Can you work these out from the model? Positions are in its coordinate system, mm. A direction names the side the tool comes from. Give positions to 0.01 mm unless a question says otherwise; leave off trailing zeros. Write each loop counter-clockwise with the first axis right and the second up, starting at its lowest first coordinate (ties: lowest second). Pieces come first, ordered by that corner, then holes. Notation, with made-up numbers: (-31, 89) -> (14, 89) arc R15 ccw to (14, 107) -> close; hole circle Ø7 at (-4, 35.5). An arc over 180 degrees is marked (long way). Answer as CSV lines item,"result". Start each with the question number.
1. I'm going to push flat-ended pins straight in: P1, Ø3, axis at y = 1.5, z = -6, coming from the -X side; P2, Ø4, axis at y = 1, z = -6.5, coming from the +X side; P3, Ø1.5, axis at x = 0, y = 0, coming from the +Z side. Where does each tip first touch, or does it pass through?
2. I need wall thicknesses on line 1 (Z direction, x = -1, y = 3); line 2 (X direction, y = -0.75, z = -2.25); line 3 (Z direction, x = -0.75, y = -1). Which ranges of each line are inside material? Lowest first, please. Write a range as [from, to].
3. If we section it at B-B on z = -3.5: Write out the boundary of the cut face in (x, y), plus the area to 3 significant figures.
4. If we section it at A-A on y = 0: Write out the boundary of the cut face in (x, z), plus the area to 3 significant figures.
5. If we section it at C-C on z = -10.25: Write out the boundary of the cut face in (x, y), plus the area to 3 significant figures.
6. On a 3-axis mill with a long thin cutter (end or side, diameter ignored), from which of +Z, -Z, +X, -X, +Y, -Y can I reach the whole of each face in a straight line? I mean faces 1 (the face through (0, 0, -14)), 2 (the face through (1.32, 2.24, -1.48)). Say none if no direction works.
7. If we mould it in two halves opening along X, with no side actions, what happens to faces 3 (the face through (-1.28, 2.26, -1.48)), 4 (the face through (0, 0, -3)), 5 (the face through (2.5, 0.1, -8.7)), 6 (the face through (0, 3, -4))? For each: pulls with the +X half, pulls with the -X half, needs draft (parallel to the pull), parting line crosses it, or undercut.
```python
from build123d import *

# Parameters (mm, degrees)
SKETCH1_R           = 4
BOSS_EXTRUDE1_DEPTH = 4
CHAMFER1_SIZE       = 0.25
CUT_EXTRUDE1_DEPTH  = 3
SKETCH3_R           = 2.5
BOSS_EXTRUDE2_DEPTH = 10
CHAMFER2_SIZE       = 0.5


with BuildPart() as part:
    # Sketch1 → Boss-Extrude1 (new body)
    with BuildSketch(Plane(origin=(0, 0, 0), x_dir=(0, 1, 0), z_dir=(0, 0, 1))):
        with Locations(Location((0, 0, 0), (0, 0, 270))):
            Circle(SKETCH1_R)
    extrude(amount=-BOSS_EXTRUDE1_DEPTH)

    # Chamfer1
    chamfer1_edges = [part.edges().sort_by_distance(p)[0] for p in [
        (-4, 0, 0),
        (-4, 0, -4),
    ]]
    chamfer(chamfer1_edges, length=CHAMFER1_SIZE)

    # Sketch2 → Cut-Extrude1 (cut)
    with BuildSketch(Plane.XY):
        Polygon((0, 3), (-2.598076211, 1.5), (-2.598076211, -1.5), (0, -3), (2.598076211, -1.5), (2.598076211, 1.5), align=None)
    extrude(amount=-CUT_EXTRUDE1_DEPTH, mode=Mode.SUBTRACT)

    # Sketch3 → Boss-Extrude2 (add)
    with BuildSketch(Plane(origin=(0, 0, -4), x_dir=(1, 0, 0), z_dir=(0, 0, -1))):
        with Locations(Location((0, 0, 0), (0, 0, 180))):
            Circle(SKETCH3_R)
    extrude(amount=BOSS_EXTRUDE2_DEPTH)

    # Chamfer2
    chamfer2_edges = [part.edges().sort_by_distance(p)[0] for p in [
        (2.5, 0, -14),
    ]]
    chamfer(chamfer2_edges, length=CHAMFER2_SIZE)


solid = part.part
```
Computed values:
1,P1,"stops at x = -2.5"
1,P2,"stops at x = 2.5"
1,P3,"stops at z = -3"
2,line 1,"z = [-4, 0]"
2,line 2,"x = [-3.93, -2.6], [2.6, 3.93]"
2,line 3,"z = [-14, -3]"
3,outline,"circle Ø8 at (0, 0)"
3,area,"50.3 mm2"
4,outline,"(-4, -3.75) -> (-3.75, -4) -> (-2.5, -4) -> (-2.5, -13.5) -> (-2, -14) -> (2, -14) -> (2.5, -13.5) -> (2.5, -4) -> (3.75, -4) -> (4, -3.75) -> (4, -0.25) -> (3.75, 0) -> (2.6, 0) -> (2.6, -3) -> (-2.6, -3) -> (-2.6, 0) -> (-3.75, 0) -> (-4, -0.25) -> close"
4,area,"66.0 mm2"
5,outline,"circle Ø5 at (0, 0)"
5,area,"19.6 mm2"
6,face 1,"-Z, +X, -X, +Y, -Y"
6,face 2,"+Z"
7,face 3,"undercut"
7,face 4,"undercut"
7,face 5,"parting line crosses it"
7,face 6,"needs draft"
